Input: part model. Units: mm. Frame: model coordinates. A direction names the side the tool comes from. Give positions to 0.01 mm unless a question says otherwise; leave off trailing zeros. Write each loop counter-clockwise with the first axis right and the second up, starting at its lowest first coordinate (ties: lowest second). Pieces come first, ordered by that corner, then holes. Notation, with made-up numbers: (88, 77.5) -> (120, 77.5) arc R22 ccw to (120, 115.5) -> close; hole circle Ø10 at (46.5, 45.5). An arc over 180 degrees is marked (long way). Return JSON: item names as keys, results as strings. Group by question number.
Item 1: Section D-D, the plane x = -7. Return loops of the section in (y, z), then the cut area to 3 significant figures.
Item 2: Set-up query: faces 1 (the face through (-4, 5, -3)), 2 (the face through (-5.535, 7.578, -3.408)). Return all of +Z, -Z, +X, -X, +Y, -Y with unobstructed straight access to the full face (end or side cutting, diameter ignored); none if empty.
Item 3: Section B-B, the plane z = -6. Return loops of the section in (x, y), then the cut area to 3 significant figures.
Item 4: Section C-C, the plane y = 7.5. Return loops of the section in (x, z), then the cut area to 3 significant figures.
Item 5: Pin query (flat end, axial travel): P1, Ø1, axis at y = 1.5, z = -5.5, coming from the +X side; P2, Ø2.5, axis at x = -3, z = -1.5, coming from the -Y side. Return the tip coordinate at first contact, or that it passes through.
Item 6: Section A-A, the plane x = -2. Return loops of the section in (y, z), then the cut area to 3 significant figures.
Item 7: Mould query, pull axis Z, two halves, no side actions, for faces 3 (the face through (-6.39, -0.15, -3.93)), 4 (the face through (-6.621, 0.153, 1.497)), 5 (the face through (-5.535, -7.643, -3.408)). Classes: released by +Z, released by -Z, zero draft, split by the parting line, or undercut.
Item 8: Line query: line 1 (Y direction, x = -2.75, z = -4.5); line 2 (X direction, y = -2.25, z = 0); line 3 (Z direction, x = -4.75, y = -3.75). Output: solid intervals per line, ascending. Write a range as [from, to].
Autodesk Inventor part; units mm, degrees
ref_plane "YZ Plane" through (0, 0, 0) normal (1, 0, 0) x (0, 1, 0)
ref_plane "XZ Plane" through (0, 0, 0) normal (0, 1, 0) x (-1, 0, 0)
ref_plane "XY Plane" through (0, 0, 0) normal (0, 0, 1) x (1, 0, 0)
sketch "Sketch1" plane through (0, 0, 0) normal (0, 1, 0) x (-1, 0, 0)
  arc A0 (1.6544, -7.3153) -> (7.3153, 1.6544) centre (0, 0) ccw
  arc A1 (1.4338, -6.3399) -> (6.3399, 1.4338) centre (0, 0) ccw
  line L0 (7.3153, 1.6544) -> (6.3399, 1.4338)
  line L1 (1.4338, -6.3399) -> (1.6544, -7.3153)
  dimension "d0" = 7.5
  dimension "d1" = 1
  dimension "d4" = 90
extrude "Extrusion1" add sketch "Sketch1" along normal mid plane 19.821
sketch "Sketch2" plane through (0, 9.9105, 0) normal (0, 1, 0) x (1, 0, 0)
  arc A0 (-1.6544, 7.3153) -> (-7.3153, -1.6544) centre (0, 0) ccw
  arc A1 (-1.1029, 4.8768) -> (-4.8768, -1.1029) centre (0, 0) ccw
  line L0 (-7.3153, -1.6544) -> (-4.8768, -1.1029)
  line L1 (-1.1029, 4.8768) -> (-1.6544, 7.3153)
  line L2 (-7.3153, -1.6544) -> (-6.3399, -1.4338)
  line L3 (-1.4338, 6.3399) -> (-1.6544, 7.3153)
  dimension "d9" = 2.5
extrude "Extrusion2" add sketch "Sketch2" along normal blind 1
mirror "Mirror1" about plane through (0, 0, 0) normal (0, 1, 0) of "Extrusion2"
ref_plane "Work Plane2" through (0, 5.3105, 0) normal (0, -1, 0) x (1, 0, 0)
sketch "Sketch3" plane through (0, 5.3105, 0) normal (0, -1, 0) x (1, 0, 0)
  arc A0 (-7.3153, 1.6544) -> (-1.6544, -7.3153) centre (0, 0) ccw
  line L0 (-7.3153, 1.6544) -> (-4.8768, 1.1029)
  arc A1 (-4.8768, 1.1029) -> (-1.1029, -4.8768) centre (0, 0) ccw
  line L1 (-1.1029, -4.8768) -> (-1.6544, -7.3153)
extrude "Extrusion3" add sketch "Sketch3" along normal blind 1
mirror "Mirror2" about plane through (0, 0, 0) normal (0, 1, 0) of "Extrusion3"
ref_plane "Work Plane3" through (-6.3399, 12.512, 1.4338) normal (-0.8457, 0, -0.5337) x (0.5337, 0, -0.8457)
sketch "Sketch4" plane through (-14.3948, 12.512, -3.6499) normal (-0.8457, 0, -0.5337) x (0.5337, 0, -0.8457)
  line L0 (3.7075, 16.0789) -> (7.5195, 16.0789) construction
  line L1 (7.5195, 16.0789) -> (7.5195, 13.4854) construction
  line L2 (7.5195, 13.4854) -> (3.7075, 13.4854) construction
  line L3 (3.7075, 13.4854) -> (3.7075, 16.0789) construction
  point P0 (4.5962, 12.512)
ref_plane "Work Plane1" through (0, 0, 0) normal (0, 1, 0) x (-1, 0, 0)
properties part number "circular_tether"
Answer below:
{
 "1": {"outline": "(-10.91, -2.69) -> (10.91, -2.69) -> (10.91, 1.58) -> (-10.91, 1.58) -> close", "area": "93.3 mm2"},
 "2": {"face 1": "+X, +Y, -Y", "face 2": "+X"},
 "3": {"outline": "(-4.5, -10.91) -> (-1.36, -10.91) -> (-1.36, -9.91) -> (-2.5, -9.91) -> (-2.5, -5.31) -> (-1.36, -5.31) -> (-1.36, -4.31) -> (-2.5, -4.31) -> (-2.5, 4.31) -> (-1.36, 4.31) -> (-1.36, 5.31) -> (-2.5, 5.31) -> (-2.5, 9.91) -> (-1.36, 9.91) -> (-1.36, 10.91) -> (-4.5, 10.91) -> close", "area": "48.2 mm2"},
 "4": {"outline": "(-7.32, 1.65) arc R7.5 ccw to (-1.65, -7.32) -> (-1.43, -6.34) arc R6.5 cw to (-6.34, 1.43) -> close", "area": "11.0 mm2"},
 "5": {"P1": "stops at x = -2.5", "P2": "passes through"},
 "6": {"outline": "(-10.91, -7.23) -> (10.91, -7.23) -> (10.91, -4.58) -> (9.91, -4.58) -> (9.91, -6.18) -> (5.31, -6.18) -> (5.31, -4.58) -> (4.31, -4.58) -> (4.31, -6.18) -> (-4.31, -6.18) -> (-4.31, -4.58) -> (-5.31, -4.58) -> (-5.31, -6.18) -> (-9.91, -6.18) -> (-9.91, -4.58) -> (-10.91, -4.58) -> close", "area": "29.2 mm2"},
 "7": {"face 3": "split by the parting line", "face 4": "released by +Z", "face 5": "undercut"},
 "8": {"line 1": "y = [-10.91, -9.91], [-5.31, -4.31], [4.31, 5.31], [9.91, 10.91]", "line 2": "x = [-7.5, -6.5]", "line 3": "z = [-5.8, -4.44]"}
}
